Check sheet for the modelled part. Datum: model origin and axes. Units: mm. Face numbers are marked on the shaded views. A direction names the side the tool comes from. Coordinates: 2 decimals unless noted, no trailing zeros. Loops run counter-clockwise (first coordinate to the right, second up) from the corner with the lowest first, then second, coordinate; pieces in that order, holes last. Notation, with made-up numbers: M 36.5,-37.5 L 89.5,-37.5 A34 cw 89.5,0.5 Z; hole C 62.25,-14 d5. An arc over 180 degrees is marked long. Answer as CSV lines item,"result". Start each with the question number.
from build123d import *

# Parameters (mm, degrees)
ESQUISSE1_R                  = 2
EXTRUSION1_DEPTH             = 17
CONG_1_R                     = 6
ESQUISSE5_R                  = 6.5
EXTRUSION3_DEPTH             = 4
EXTRUSION3_DIRECTION_2_REACH = 74.726
ESQUISSE6_R                  = 7.5
EXTRUSION4_DEPTH             = 30
ESQUISSE7_R                  = 4.5
EXTRUSION5_DEPTH             = 15
CHANFREIN2_SIZE              = 3
ESQUISSE8_R                  = 3
EXTRUSION6_DEPTH             = 15
CHANFREIN3_SIZE              = 1
EXTRUSION7_DEPTH             = 0.5
ESQUISSE10_R                 = 2.5
EXTRUSION8_DEPTH             = 0.5


with BuildPart() as part:
    # Esquisse1 → Extrusion1 (new body)
    with BuildSketch(Plane.XY):
        Polygon((0, 50), (0, 15), (17, 0), (50, 0), (50, 44.696699141), (44.696699141, 50), align=None)
        with Locations((4, 15)):
            Circle(ESQUISSE1_R, mode=Mode.SUBTRACT)
        with BuildLine():
            Line((2, 43), (2, 46))
            ThreePointArc((2, 46), (4, 48), (6, 46))
            Line((6, 46), (6, 43))
            ThreePointArc((6, 43), (4, 41), (2, 43))
        make_face(mode=Mode.SUBTRACT)
        with BuildLine():
            Line((40, 6), (46, 6))
            ThreePointArc((46, 6), (48, 4), (46, 2))
            Line((46, 2), (40, 2))
            ThreePointArc((40, 2), (38, 4), (40, 6))
        make_face(mode=Mode.SUBTRACT)
    extrude(amount=EXTRUSION1_DEPTH)

    # Congé1
    cong_1_edges = [part.edges().sort_by_distance(p)[0] for p in [
        (47.348349571, 47.348349571, 17),
        (47.348349571, 47.348349571, 0),
    ]]
    fillet(cong_1_edges, radius=CONG_1_R)

    # Esquisse5 → Extrusion3 (add)
    with BuildSketch(Plane.XZ):
        with Locations(Location((8.5, 8.5, 0), (0, 0, 270))):
            Circle(ESQUISSE5_R)
    extrude(amount=EXTRUSION3_DEPTH)

    # Esquisse5 → Extrusion3 direction 2 (add, up to next)
    with BuildSketch(Plane.XZ, mode=Mode.PRIVATE) as extrusion3_direction_2_sk1:
        with Locations(Location((8.5, 8.5, 0), (0, 0, 270))):
            Circle(ESQUISSE5_R)
    extrusion3_direction_2_tool1 = extrude(extrusion3_direction_2_sk1.sketch, amount=-EXTRUSION3_DIRECTION_2_REACH, mode=Mode.PRIVATE) - part.part
    add(extrusion3_direction_2_tool1.solids().sort_by_distance((8.5, 0, 8.5))[0])

    # Esquisse6 → Extrusion4 (add)
    with BuildSketch(Plane.XZ.offset(4)):
        with Locations(Location((8.5, 8.5, 0), (0, 0, 270))):
            Circle(ESQUISSE6_R)
    extrude(amount=EXTRUSION4_DEPTH)

    # Esquisse7 → Extrusion5 (add)
    with BuildSketch(Plane.XZ.offset(34)):
        with Locations(Location((8.5, 8.5, 0), (0, 0, 270))):
            Circle(ESQUISSE7_R)
    extrude(amount=EXTRUSION5_DEPTH)

    # Chanfrein2
    chanfrein2_edges = [part.edges().sort_by_distance(p)[0] for p in [
        (8.5, -34, 13),
    ]]
    chamfer(chanfrein2_edges, length=CHANFREIN2_SIZE - 0.0001)  # a hair under: the kernel refuses the full size

    # Esquisse8 → Extrusion6 (add)
    with BuildSketch(Plane.XZ.offset(49)):
        with Locations(Location((8.5, 8.5, 0), (0, 0, 270))):
            Circle(ESQUISSE8_R)
    extrude(amount=EXTRUSION6_DEPTH)

    # Chanfrein3
    chanfrein3_edges = [part.edges().sort_by_distance(p)[0] for p in [
        (8.5, -49, 11.5),
    ]]
    chamfer(chanfrein3_edges, length=CHANFREIN3_SIZE)

    # Esquisse9 → Extrusion7 (cut)
    with BuildSketch(Plane(origin=(50, 0, 0), x_dir=(0, 0, -1), z_dir=(1, 0, 0))):
        with BuildLine():
            Line((-15.5, 14), (-15.5, 36.196699141))
            ThreePointArc((-15.5, 36.196699141), (-8.5, 43.196699141), (-1.5, 36.196699141))
            Line((-1.5, 36.196699141), (-1.5, 14))
            ThreePointArc((-1.5, 14), (-8.5, 7), (-15.5, 14))
        make_face()
    extrude(amount=-EXTRUSION7_DEPTH, mode=Mode.SUBTRACT)

    # Esquisse10 → Extrusion8 (cut)
    with BuildSketch(Plane(origin=(0, 50, 0), x_dir=(1, 0, 0), z_dir=(0, 1, 0))):
        with BuildLine():
            Line((14, -1.5), (36.196699141, -1.5))
            ThreePointArc((36.196699141, -1.5), (43.196699141, -8.5), (36.196699141, -15.5))
            Line((36.196699141, -15.5), (14, -15.5))
            ThreePointArc((14, -15.5), (7, -8.5), (14, -1.5))
        make_face()
        with Locations(Location((14, -8.5, 0), (0, 0, 180))):
            Circle(ESQUISSE10_R, mode=Mode.SUBTRACT)
        with Locations(Location((22.348349571, -8.5, 0), (0, 0, 180))):
            Circle(ESQUISSE10_R, mode=Mode.SUBTRACT)
    extrude(amount=-EXTRUSION8_DEPTH, mode=Mode.SUBTRACT)


solid = part.part
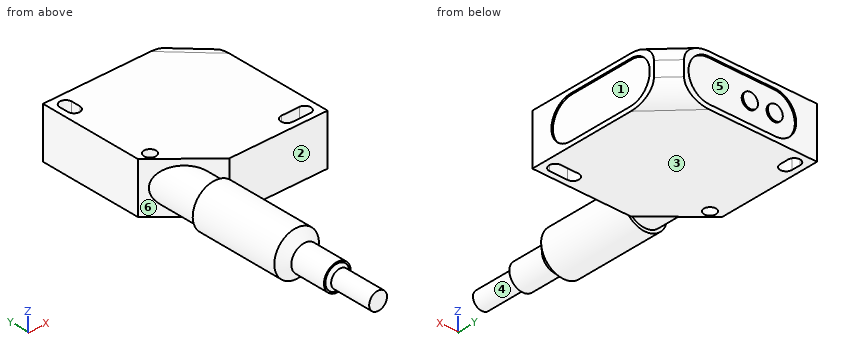
Item 1: Sectioned sample at B-B, the plane y = -8.5. Record the boundary of the cut face in (x, z), and give its area (3 significant figures).
Item 2: Sectioned sample at D-D, the plane z = 7.25. Give the number of separate pieces and of enclosed holes in the cut face, and give its area (3 significant figures).
Item 3: Sectioned sample at A-A, the plane x = 31. Record the boundary of the cut face in (y, z).
Item 4: Material ranges on line 1 (Y direction, x = 4, z = 10.75); line 2 (Y direction, x = 4, z = 5); line 3 (X direction, y = 39.5, z = 12), recorded low to high. Write a range as from..to.
Item 5: Release check for a two-part mould opening along Y. For the marked faces 1, 2 and 3 record: released by +Y, released by -Y, zero draft, split by the parting line, or undercut.
Item 6: Go/stop test with flat-tipped pins: pin 1 (4 mm diameter, centred on x = 26, z = 14.5, fed in from -Y); pin 2 (1.5 mm diameter, centred on y = 22, z = 13.5, fed in from +X); pin 3 (2 mm diameter, centred on y = -14.5, z = 6, fed in from -X); pin 4 (3 mm diameter, centred on x = 4, y = 15, fed in from +Z). Record where each tip stops, or that it passes through.
Item 7: Set-up check for the marked faces 4, 5 and 6: record each of +Z, -Z, +X, -X, +Y, -Y from which the full face is reachable in a straight line by a thin tool's end or side.
Reply:
1,outline,"C 8.5,8.5 d15"
1,area,"177 mm²"
2,separate pieces,"1"
2,enclosed holes,"3"
2,area,"3,070 mm²"
3,outline,"M 0,0 L 50,0 L 50,1.5 L 49.5,1.5 L 49.5,15.5 L 50,15.5 L 50,17 L 0,17 Z"
4,line 1,"-36.47..13, 17..41, 48..50"
4,line 2,"-35.8..13, 17..41, 48..50"
4,line 3,"0..49.5"
5,face 1,"undercut"
5,face 2,"released by -Y"
5,face 3,"zero draft"
6,pin 1,"y = 0"
6,pin 2,"x = 49.5"
6,pin 3,"x = 1.15"
6,pin 4,"through"
7,face 4,"-Y"
7,face 5,"+Y"
7,face 6,"none"
